from build123d import *

# Parameters (mm, degrees)
SKETCH1_W           = 914.4
SKETCH1_H           = 406.4
SKETCH1_W_2         = 876.3
SKETCH1_H_2         = 368.3
BOSS_EXTRUDE1_DEPTH = 19.05
FILLET1_R           = 1.016
FILLET2_R           = 1.016


with BuildPart() as part:
    # Sketch1 → Boss-Extrude1 (new body)
    with BuildSketch(Plane(origin=(0, 0, 0), x_dir=(1, 0, 0), z_dir=(0, 1, 0))):
        Rectangle(SKETCH1_W, SKETCH1_H)
        Rectangle(SKETCH1_W_2, SKETCH1_H_2, mode=Mode.SUBTRACT)
    extrude(amount=BOSS_EXTRUDE1_DEPTH)

    # Fillet1
    fillet1_edges = [part.edges().sort_by_distance(p)[0] for p in [
        (-457.2, 19.05, 0),
        (438.15, 0, 0),
        (0, 0, -184.15),
        (-438.15, 0, 0),
        (0, 0, 184.15),
        (438.15, 19.05, 0),
        (0, 19.05, 203.2),
        (0, 19.05, -184.15),
        (-438.15, 19.05, 0),
        (0, 19.05, 184.15),
        (457.2, 19.05, 0),
        (0, 0, 203.2),
        (-457.2, 0, 0),
        (0, 0, -203.2),
        (457.2, 0, 0),
        (0, 19.05, -203.2),
    ]]
    fillet(fillet1_edges, radius=FILLET1_R)

    # Fillet2
    # the kernel refuses this fillet: 1.016 mm, written as the material it takes off along each edge
    with BuildSketch(Plane(origin=(456.184, 1.016, 202.184), x_dir=(1, 0, 0), z_dir=(0, 0, 1))) as fillet2_piece_1_section:
        Polygon((0, 0), (FILLET2_R * 1.02, 0), (FILLET2_R * 1.02, -FILLET2_R * 1.02), (0, -FILLET2_R * 1.02), align=None)
    fillet2_piece_1 = extrude(amount=FILLET2_R * 1.02, mode=Mode.PRIVATE)
    fillet2_piece_1 = fillet2_piece_1 - Plane(origin=(456.184, 1.016, 202.184), x_dir=(-0.7071067811865475, 0.7071067811865475, 0), z_dir=(0, 0, 1)) * Sphere(FILLET2_R, mode=Mode.PRIVATE)
    add(fillet2_piece_1, mode=Mode.SUBTRACT)
    with BuildSketch(Plane(origin=(-456.184, 1.016, 202.184), x_dir=(-1, 0, 0), z_dir=(0, 0, 1))) as fillet2_piece_2_section:
        Polygon((0, 0), (FILLET2_R * 1.02, 0), (FILLET2_R * 1.02, FILLET2_R * 1.02), (0, FILLET2_R * 1.02), align=None)
    fillet2_piece_2 = extrude(amount=FILLET2_R * 1.02, mode=Mode.PRIVATE)
    fillet2_piece_2 = fillet2_piece_2 - Plane(origin=(-456.184, 1.016, 202.184), x_dir=(0.7071067811865475, 0.7071067811865475, 0), z_dir=(0, 0, 1)) * Sphere(FILLET2_R, mode=Mode.PRIVATE)
    add(fillet2_piece_2, mode=Mode.SUBTRACT)
    with BuildSketch(Plane(origin=(456.184, 1.016, -202.184), x_dir=(0, 0, -1), z_dir=(1, 0, 0))) as fillet2_piece_3_section:
        Polygon((0, 0), (FILLET2_R * 1.02, 0), (FILLET2_R * 1.02, -FILLET2_R * 1.02), (0, -FILLET2_R * 1.02), align=None)
    fillet2_piece_3 = extrude(amount=FILLET2_R * 1.02, mode=Mode.PRIVATE)
    fillet2_piece_3 = fillet2_piece_3 - Plane(origin=(456.184, 1.016, -202.184), x_dir=(0, 0.7071067811865475, 0.7071067811865475), z_dir=(1, 0, 0)) * Sphere(FILLET2_R, mode=Mode.PRIVATE)
    add(fillet2_piece_3, mode=Mode.SUBTRACT)
    with BuildSketch(Plane(origin=(-456.184, 1.016, -202.184), x_dir=(0, 0, -1), z_dir=(-1, 0, 0))) as fillet2_piece_4_section:
        Polygon((0, 0), (FILLET2_R * 1.02, 0), (FILLET2_R * 1.02, FILLET2_R * 1.02), (0, FILLET2_R * 1.02), align=None)
    fillet2_piece_4 = extrude(amount=FILLET2_R * 1.02, mode=Mode.PRIVATE)
    fillet2_piece_4 = fillet2_piece_4 - Plane(origin=(-456.184, 1.016, -202.184), x_dir=(0, 0.7071067811865475, 0.7071067811865475), z_dir=(-1, 0, 0)) * Sphere(FILLET2_R, mode=Mode.PRIVATE)
    add(fillet2_piece_4, mode=Mode.SUBTRACT)
    with BuildSketch(Plane(origin=(-456.184, 18.034, -202.184), x_dir=(0, 0, -1), z_dir=(-1, 0, 0))) as fillet2_piece_5_section:
        Polygon((0, 0), (FILLET2_R * 1.02, 0), (FILLET2_R * 1.02, -FILLET2_R * 1.02), (0, -FILLET2_R * 1.02), align=None)
    fillet2_piece_5 = extrude(amount=FILLET2_R * 1.02, mode=Mode.PRIVATE)
    fillet2_piece_5 = fillet2_piece_5 - Plane(origin=(-456.184, 18.034, -202.184), x_dir=(0, -0.7071067811865475, 0.7071067811865475), z_dir=(-1, 0, 0)) * Sphere(FILLET2_R, mode=Mode.PRIVATE)
    add(fillet2_piece_5, mode=Mode.SUBTRACT)
    with BuildSketch(Plane(origin=(456.184, 18.034, -202.184), x_dir=(0, 0, -1), z_dir=(1, 0, 0))) as fillet2_piece_6_section:
        Polygon((0, 0), (FILLET2_R * 1.02, 0), (FILLET2_R * 1.02, FILLET2_R * 1.02), (0, FILLET2_R * 1.02), align=None)
    fillet2_piece_6 = extrude(amount=FILLET2_R * 1.02, mode=Mode.PRIVATE)
    fillet2_piece_6 = fillet2_piece_6 - Plane(origin=(456.184, 18.034, -202.184), x_dir=(0, -0.7071067811865475, 0.7071067811865475), z_dir=(1, 0, 0)) * Sphere(FILLET2_R, mode=Mode.PRIVATE)
    add(fillet2_piece_6, mode=Mode.SUBTRACT)
    with BuildSketch(Plane(origin=(-456.184, 18.034, 202.184), x_dir=(-1, 0, 0), z_dir=(0, 0, 1))) as fillet2_piece_7_section:
        Polygon((0, 0), (FILLET2_R * 1.02, 0), (FILLET2_R * 1.02, -FILLET2_R * 1.02), (0, -FILLET2_R * 1.02), align=None)
    fillet2_piece_7 = extrude(amount=FILLET2_R * 1.02, mode=Mode.PRIVATE)
    fillet2_piece_7 = fillet2_piece_7 - Plane(origin=(-456.184, 18.034, 202.184), x_dir=(0.7071067811865475, -0.7071067811865475, 0), z_dir=(0, 0, 1)) * Sphere(FILLET2_R, mode=Mode.PRIVATE)
    add(fillet2_piece_7, mode=Mode.SUBTRACT)
    with BuildSketch(Plane(origin=(456.184, 18.034, 202.184), x_dir=(1, 0, 0), z_dir=(0, 0, 1))) as fillet2_piece_8_section:
        Polygon((0, 0), (FILLET2_R * 1.02, 0), (FILLET2_R * 1.02, FILLET2_R * 1.02), (0, FILLET2_R * 1.02), align=None)
    fillet2_piece_8 = extrude(amount=FILLET2_R * 1.02, mode=Mode.PRIVATE)
    fillet2_piece_8 = fillet2_piece_8 - Plane(origin=(456.184, 18.034, 202.184), x_dir=(-0.7071067811865475, -0.7071067811865475, 0), z_dir=(0, 0, 1)) * Sphere(FILLET2_R, mode=Mode.PRIVATE)
    add(fillet2_piece_8, mode=Mode.SUBTRACT)
    with BuildSketch(Plane(origin=(-457.2, 1.016, -203.2), x_dir=(0, 0, 1), z_dir=(0, 1, 0)), Plane(origin=(-457.2, 1.016, 203.2), x_dir=(1, 0, 0), z_dir=(0, 1, 0))) as fillet2_piece_9:
        with BuildLine():
            CenterArc((FILLET2_R, FILLET2_R), FILLET2_R, 180, 90)
            Line((0, FILLET2_R), (0, 0))
            Line((0, 0), (FILLET2_R, 0))
        make_face()
    extrude(amount=17.018, mode=Mode.SUBTRACT)
    with BuildSketch(Plane(origin=(457.2, 1.016, -203.2), x_dir=(0, 0, 1), z_dir=(0, 1, 0)), Plane(origin=(457.2, 1.016, 203.2), x_dir=(-1, 0, 0), z_dir=(0, 1, 0))) as fillet2_piece_10:
        with BuildLine():
            CenterArc((FILLET2_R, -FILLET2_R), FILLET2_R, 90, 90)
            Line((0, -FILLET2_R), (0, 0))
            Line((0, 0), (FILLET2_R, 0))
        make_face()
    extrude(amount=17.018, mode=Mode.SUBTRACT)


solid = part.part
Could you check a few things on this model? Use its own coordinates, in mm. A direction names the side the tool comes from. Round coordinates to 2 decimals unless told otherwise and drop trailing zeros. Write each loop counter-clockwise with the first axis right and the second up, starting at its lowest first coordinate (ties: lowest second). Pieces come first, ordered by that corner, then holes. Notation, with made-up numbers: (87, -9) - (116, -9) arc R18 ccw to (116, 3) - close; hole circle Ø5 at (11, -28.75). An arc over 180 degrees is marked (long way). Put each result on its own line as item: value. Start each with the question number.
(1) For faces 1 (the flat face through (-438.15, 9, 3)), 2 (the flat face through (457.2, 9, 3)), which set-ups out of +Z, -Z, +X, -X, +Y, -Y let a thin tool reach every point of the face, with its end or its side?
(2) I need wall thicknesses on probe 1 along X at (y, z) = (1, 82.5); probe 2 along Z at (x, y) = (366, 2.5). Which ranges of each line are inside material? Lowest first, please.
(3) Thinking about a two-plate mould opening in Z: for faces 3 (the flat face through (438.15, 9, 3)), 4 (the flat face through (-6, 9, 203.2)), 5 (the flat face through (-6, 9, 184.15)), 6 (the flat face through (-457.2, 9, 3)), which applies, released by +Z, released by -Z, zero draft, split by the parting line, or undercut?
(4) I want a section at B-B, the plane z = 113. Please give me the cut outline in (x, y), plus the area to 3 significant figures.
(5) I want a section at C-C, the plane y = 8.75. Please give me the cut outline in (x, z), plus the area to 3 significant figures.
(6) I want a section at A-A, the plane x = -0.5. Please give me the cut outline in (y, z).
Here are the results:
1. face 1: +Y, -Y
1. face 2: +Z, -Z, +X, +Y, -Y
2. probe 1: x = -457.2 to -438.15, 438.15 to 457.2
2. probe 2: z = -203.2 to -184.15, 184.15 to 203.2
3. face 3: undercut
3. face 4: released by +Z
3. face 5: undercut
3. face 6: zero draft
4. outline: (-457.2, 1.02) arc R1.02 ccw to (-456.18, 0) - (-439.17, 0) arc R1.02 ccw to (-438.15, 1.02) - (-438.15, 18.03) arc R1.02 ccw to (-439.17, 19.05) - (-456.18, 19.05) arc R1.02 ccw to (-457.2, 18.03) - close; (438.15, 1.02) arc R1.02 ccw to (439.17, 0) - (456.18, 0) arc R1.02 ccw to (457.2, 1.02) - (457.2, 18.03) arc R1.02 ccw to (456.18, 19.05) - (439.17, 19.05) arc R1.02 ccw to (438.15, 18.03) - close
4. area: 724 mm^2
5. outline: (-457.2, -202.18) arc R1.02 ccw to (-456.18, -203.2) - (456.18, -203.2) arc R1.02 ccw to (457.2, -202.18) - (457.2, 202.18) arc R1.02 ccw to (456.18, 203.2) - (-456.18, 203.2) arc R1.02 ccw to (-457.2, 202.18) - close; hole (-438.15, -184.15) - (438.15, -184.15) - (438.15, 184.15) - (-438.15, 184.15) - close
5. area: 48,900 mm^2
6. outline: (0, -202.18) arc R1.02 ccw to (1.02, -203.2) - (18.03, -203.2) arc R1.02 ccw to (19.05, -202.18) - (19.05, -185.17) arc R1.02 ccw to (18.03, -184.15) - (1.02, -184.15) arc R1.02 ccw to (0, -185.17) - close; (0, 185.17) arc R1.02 ccw to (1.02, 184.15) - (18.03, 184.15) arc R1.02 ccw to (19.05, 185.17) - (19.05, 202.18) arc R1.02 ccw to (18.03, 203.2) - (1.02, 203.2) arc R1.02 ccw to (0, 202.18) - close
